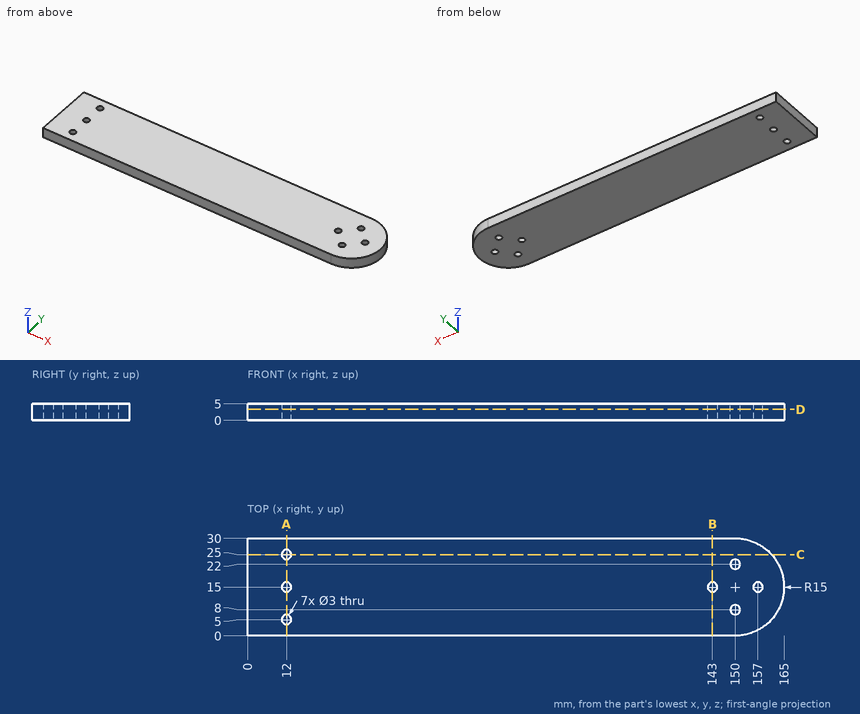
Answer from the drawing. Dimensions are ordinates in mm from the lowest x, y and z of the part. Coordinates: 2 decimals unless noted, no trailing zeros. Write each loop counter-clockwise with the first axis right and the second up, starting at its lowest first coordinate (ties: lowest second). Pieces come first, ordered by that corner, then holes. Notation, with made-up numbers: M 58,15.5 L 77,15.5 A21 ccw 77,39.5 Z; hole C 54,35.25 d2. An arc over 180 degrees is marked long. Use one line per item in the form item = value. Start each with the question number.
1. The part is cut by section A-A (x = 12). Give the vertices of the cut face in (y, z), plus the area to 3 significant figures.
2. Straight lines are drawn through the part: probe 1 along Y at (x, z) = (12, 3.55); probe 2 along Y at (x, z) = (157, 1.3); probe 3 along X at (y, z) = (25.25, 1.25). For each, find the intervals that lie inside material, in ascending order. Write a range as from..to.
3. The part is cut by section B-B (x = 143). Give the vertices of the cut face in (y, z), plus the area to 3 significant figures.
4. The part is cut by section C-C (y = 25). Give the vertices of the cut face in (x, z).
5. Each of these flat-tipped pins is pushed along its axis until it touches: P1, Ø2, axis at y = 20, z = 1, coming from the +X side; P2, Ø2, axis at y = 7, z = 4.5, coming from the +X side. Where does it stop, or does it pass through?
6. The part is cut by section D-D (z = 3.35). Give the vertices of the cut face in (x, y).
Evaluation:
q1.outline = M 0,0 L 3.5,0 L 3.5,5 L 0,5 Z; M 6.5,0 L 13.5,0 L 13.5,5 L 6.5,5 Z; M 16.5,0 L 23.5,0 L 23.5,5 L 16.5,5 Z; M 26.5,0 L 30,0 L 30,5 L 26.5,5 Z
q1.area = 105 mm^2
q2.probe_1 = 0..3.5, 6.5..13.5, 16.5..23.5, 26.5..30
q2.probe_2 = 1.73..13.5, 16.5..28.27
q2.probe_3 = 0..10.52, 13.48..160.95
q3.outline = M 0,0 L 13.5,0 L 13.5,5 L 0,5 Z; M 16.5,0 L 30,0 L 30,5 L 16.5,5 Z
q3.area = 135 mm^2
q4.outline = M 0,0 L 10.5,0 L 10.5,5 L 0,5 Z; M 13.5,0 L 161.18,0 L 161.18,5 L 13.5,5 Z
q5.P1 = 164.46
q5.P2 = 163.27
q6.outline = M 0,0 L 150,0 A15 ccw 150,30 L 0,30 Z; hole C 12,5 d3; hole C 12,15 d3; hole C 12,25 d3; hole C 143,15 d3; hole C 150,8 d3; hole C 150,22 d3; hole C 157,15 d3
